```python
from build123d import *

# Parameters (mm, degrees)
F0_W     = 40
F0_H     = 40
F1_DEPTH = 20
F5_DEPTH = 16.3309316186
F7_DEPTH = 5
F9_DEPTH = 15


# Not quite as in the source:
# - a pattern or mirror of a feature is missing from the dataset's text; its kind, count and spacing are read off the source's solid


with BuildPart() as f1:
    # F0 (on Right) → F1 (new body, symmetric)
    with BuildSketch(Plane.YZ):
        with Locations((20, 20)):
            Rectangle(F0_W, F0_H)
    extrude(amount=F1_DEPTH, both=True)

    # F4 (on 3pt) → F5 (cut, through all)
    with BuildSketch(Plane(origin=(13.3333333333, -6.6666666667, 6.6666666667), x_dir=(-0.3651483717, -0.9128709292, -0.1825741858), z_dir=(-0.8164965809, 0.4082482905, -0.4082482905))):
        Polygon((-7.3029674334, -8.94427191), (-7.3029674334, 35.77708764), (-51.1207720338, 26.83281573), align=None)
    f5 = extrude(amount=-F5_DEPTH, mode=Mode.SUBTRACT)

    # F5_copies: F5 across plane
    add(f5.mirror(Plane(origin=(0, 0, 0), x_dir=(0, 0, -1), z_dir=(-1, 0, 0))), mode=Mode.SUBTRACT)

    # F6 (on Right) → F7 (cut, symmetric)
    with BuildSketch(Plane.YZ):
        Polygon((0, 10), (0, 0), (40, 0), align=None)
    extrude(amount=F7_DEPTH, both=True, mode=Mode.SUBTRACT)

    # F8 (on face) → F9 (cut)
    with BuildSketch(Plane.YZ.offset(20)):
        Polygon((30, 40), (10, 40), (0, 30), (20, 30), align=None)
    f9 = extrude(amount=-F9_DEPTH, mode=Mode.SUBTRACT)

    # F9_copies: F9 across plane
    add(f9.mirror(Plane(origin=(0, 0, 0), x_dir=(0, 0, -1), z_dir=(-1, 0, 0))), mode=Mode.SUBTRACT)


solid = f1.part
```
Can you work these out from the model? Positions are in its coordinate system, mm. A direction names the side the tool comes from. Give positions to 0.01 mm unless a question says otherwise; leave off trailing zeros. Loops run counter-clockwise (first coordinate to the right, second up) from the corner with the lowest first, then second, coordinate; pieces in that order, holes last. Notation, with made-up numbers: M -28,82 L 28,82 A21 cw 28,93 Z; hole C 14.5,18.25 d4. An arc over 180 degrees is marked long. One line per question, with ' | ' between items. Start each with the question number.
Q1. If we section it at B-B (x = 7): Please give me the cut outline in (y, z).
Q2. If we section it at D-D (z = 3): Please give me the cut outline in (x, y), plus the area to 3 significant figures.
Q3. For pin 1 Ø8 at (y, z) = (17.5, 33) entering from -X; pin 2 Ø3 at (x, y) = (-9.5, 15) entering from +Z; pin 3 Ø5 at (y, z) = (13.5, 35.5) entering from +X, each with a flat end and sliding along its axis, tell me the tip position at first contact or that it passes through.
Q4. If I drill on line 1 (X direction, y = 23.5, z = 4); line 2 (Z direction, x = 5.5, y = 20); line 3 (X direction, y = 17, z = 37), over which ranges is the centre line in solid material (lowest first)? Write a range as from..to.
Q5. If we section it at C-C (z = 32): Please give me the cut outline in (x, y).
Q6. If we section it at A-A (y = 25): Please give me the cut outline in (x, z), plus the area to 3 significant figures.
Q7. If we mould it in two halves opening along X, with no side actions, what happens to faces 6 (the flat face through (-16, 16, 24)), 7 (the flat face through (0, 29, 40)), 8 (the flat face through (-5, 11, 3))? For each: +X half, -X half, draft (parallel to the pull), parting line (faces both ways), or undercut.
Q8. For faces 1 (the flat face through (8, 14, 30)), 2 (the flat face through (-12, 20, 0)), 3 (the flat face through (5, 11, 3)), 4 (the flat face through (-20, 29, 11)), 5 (the flat face through (-8, 14, 30)), which set-ups out of +Z, -Z, +X, -X, +Y, -Y let a thin tool reach every point of the face, with its end or its side?
Computed:
1) outline: M 0,0 L 40,0 L 40,40 L 30,40 L 20,30 L 4,30 L 0,26 Z
2) outline: M -20,3 L -18.5,0 L -5,0 L -5,28 L 5,28 L 5,0 L 18.5,0 L 20,3 L 20,40 L -20,40 Z | area: 1,320 mm²
3) pin 1: stops at x = -15.08 | pin 2: stops at z = 30 | pin 3: stops at x = 5
4) line 1: x = -20..-5, 5..20 | line 2: z = 0..30 | line 3: x = -5..5
5) outline: M -20,32 L -15,22 L -5,22 L -5,2 L -4,0 L 4,0 L 5,2 L 5,22 L 15,22 L 20,32 L 20,40 L -20,40 Z
6) outline: M -20,0 L -5,0 L -5,3.75 L 5,3.75 L 5,0 L 20,0 L 20,25 L 15,35 L 5,35 L 5,40 L -5,40 L -5,35 L -15,35 L -20,25 Z | area: 1,360 mm²
7) face 6: -X half | face 7: draft | face 8: undercut
8) face 1: +Z, +X, -Y | face 2: -Z, +X, -X, +Y, -Y | face 3: -Z, -Y | face 4: +Z, -Z, -X, +Y, -Y | face 5: +Z, -X, -Y
